Solid Edge part; units mm, degrees
sketch "Sketch1" plane through (0, 0, 0) normal (0, 0, 1) x (1, 0, 0)
  circle A0 centre (0, 0) radius 1.5
extrude "Protrusion1" add sketch "Sketch1" along normal blind 14
sketch "Sketch2" plane through (0, 0, 14) normal (0, 0, 1) x (1, 0, 0)
  circle A0 centre (0, 0) radius 2.5
extrude "Head" add sketch "Sketch2" along normal blind 1
fillet "Round___Head" radius 0.5 1 edges at (-2.5, 0, 15)
sketch "Sketch3" plane through (0, 0, 15) normal (0, 0, 1) x (1, 0, 0)
  line L0 (-0.5, -2.4495) -> (-0.5, 2.4495)
  line L1 (0.5, 2.4495) -> (0.5, -2.4495)
  arc A0 (0.5, -2.4495) -> (-0.5, -2.4495) centre (0, 0) cw
extrude "Cutout___Head" cut sketch "Sketch3" against normal blind 0.5 material side at (-0.45, 0, 15)
cosmetic_thread "Thread1"
properties material "Stainless Steel, 420"
Input: part model. Units: mm. Frame: model coordinates. A direction names the side the tool comes from. Round coordinates to 2 decimals unless told otherwise and drop trailing zeros. Loops run counter-clockwise (first coordinate to the right, second up) from the corner with the lowest first, then second, coordinate; pieces in that order, holes last. Notation, with made-up numbers: (74.5, -28) -> (91.5, -28) arc R29 ccw to (91.5, 7) -> close; hole circle Ø9 at (-7, -7.5). An arc over 180 degrees is marked (long way). Answer as a JSON object with one key per item and string values. Group by question number.
1) Draft query along X for faces 1 (the flat face through (2, 0, 14)), 2 (the cylindrical face through (-0.54, 2.44, 14.25)), 3 (the flat face through (0, 0, 14.5)). Return one class per face: +X half, -X half, draft (parallel to the pull), parting line (faces both ways), or undercut.
2) Section query B-B on x = 0. Output: boundary loops of the cut face in (y, z), plus the area to 3 significant figures.
3) Reachability of faces 4 (the flat face through (1, 0, 15)), 5 (the cylindrical face through (-1.5, -0.07, 6.9)) from +Z, -Z, +X, -X, +Y, -Y: full face, straight path, thin tool, end or side. Return the list, or none.
4) Pin query (flat end, axial travel): pin 1 (1.5 mm diameter, centred on x = 1.5, z = 13.5, fed in from +Y). Return the tip coordinate at first contact, or that it passes through.
5) Section query C-C on z = 8.75. Output: boundary loops of the cut face in (x, y), plus the area to 3 significant figures.
6) Ray query, L1, parallel to Z at x = -0.75, y = 1.9; L2, parallel to Z at x = -0.35, y = -0.75; L3, parallel to Y at x = -0.05, z = 1.75. Return the intervals inside material, ascending.
7) Section query A-A on y = 0. Output: boundary loops of the cut face in (x, z), plus the area to 3 significant figures.
Reply:
{
 "1": {"face 1": "draft", "face 2": "parting line", "face 3": "undercut"},
 "2": {"outline": "(-2.5, 14) -> (-1.5, 14) -> (-1.5, 0) -> (1.5, 0) -> (1.5, 14) -> (2.5, 14) -> (2.5, 14.5) -> (-2.5, 14.5) -> close", "area": "44.5 mm2"},
 "3": {"face 4": "+Z, +X, -X, +Y, -Y", "face 5": "-Z"},
 "4": {"pin 1": "stops at y = 2.32"},
 "5": {"outline": "circle Ø3 at (0, 0)", "area": "7.07 mm2"},
 "6": {"L1": "z = 14 to 15", "L2": "z = 0 to 14.5", "L3": "y = -1.5 to 1.5"},
 "7": {"outline": "(-2.5, 14) -> (-1.5, 14) -> (-1.5, 0) -> (1.5, 0) -> (1.5, 14) -> (2.5, 14) -> (2.5, 14.5) arc R0.5 ccw to (2, 15) -> (0.5, 15) -> (0.5, 14.5) -> (-0.5, 14.5) -> (-0.5, 15) -> (-2, 15) arc R0.5 ccw to (-2.5, 14.5) -> close", "area": "46.4 mm2"}
}
